Could you check a few things on this model? Use its own coordinates, in mm. A direction names the side the tool comes from. Give positions to 0.01 mm unless a question says otherwise; leave off trailing zeros. Write each loop counter-clockwise with the first axis right and the second up, starting at its lowest first coordinate (ties: lowest second). Pieces come first, ordered by that corner, then holes. Notation, with made-up numbers: M 83.5,28.25 L 103.5,28.25 A17 cw 103.5,36.25 Z; hole C 3,40 d1. An arc over 180 degrees is marked long. Write each question's results on one line, items separated by ' | '. Start each with the question number.
from build123d import *

# Parameters (mm, degrees)
F0_W          = 15.875
F0_H          = 50.8
F1_DEPTH      = 6.35
F2_W          = 31.75
F2_H          = 8.6
F2_R          = 1.75
F3_DEPTH      = 3.175
F3_DEPTH_BACK = 6.35
F4_R          = 4.7625
F5_DEPTH      = 2.54
F6_SIZE       = 2.54
F8_DEPTH      = 5.08
F9_R          = 3.81
F11_DEPTH     = 3.175
F12_SIZE      = 3.17499


# Not quite as in the source:
# - a fillet or chamfer is up to 0.001 mm smaller than in the source, because OpenCascade refuses the exact size


with BuildPart() as f1:
    # F0 (on Top) → F1 (new body)
    with BuildSketch(Plane.XY):
        Rectangle(F0_W, F0_H)
        with BuildLine():
            ThreePointArc((-3.175, -18.058110271), (0.0514516208, -14.8835271912), (3.1733324288, -18.161))
            Line((3.1733324288, -18.161), (3.1733324288, -19.431))
            ThreePointArc((3.1733324288, -19.431), (-0.053119192, -22.6055830798), (-3.175, -19.328110271))
            Line((-3.175, -19.328110271), (-3.175, -18.058110271))
        make_face(mode=Mode.SUBTRACT)
        with BuildLine():
            ThreePointArc((3.1733324288, 18.161), (0.0514516208, 14.8835271912), (-3.175, 18.058110271))
            Line((-3.175, 18.058110271), (-3.175, 19.328110271))
            ThreePointArc((-3.175, 19.328110271), (-0.053119192, 22.6055830798), (3.1733324288, 19.431))
            Line((3.1733324288, 19.431), (3.1733324288, 18.161))
        make_face(mode=Mode.SUBTRACT)
    extrude(amount=F1_DEPTH)

    # F2 (on face) → F3 (join, two sides)
    with BuildSketch(Plane.XY.offset(6.35)) as f3_sk:
        with Locations((0, 9.525)):
            Rectangle(F2_W, F2_H)
        with Locations((-10.795, 9.525)):
            Circle(F2_R, mode=Mode.SUBTRACT)
        with Locations((10.795, 9.525)):
            Circle(F2_R, mode=Mode.SUBTRACT)
    extrude(amount=F3_DEPTH)
    extrude(f3_sk.sketch, amount=-F3_DEPTH_BACK)

    # F4 (on face) → F5 (cut)
    with BuildSketch(Plane.XY.offset(6.35)):
        with Locations((0, -18.796)):
            Circle(F4_R)
        with Locations((0, 18.796)):
            Circle(F4_R)
    extrude(amount=-F5_DEPTH, mode=Mode.SUBTRACT)

    # F6
    f6_edges = [f1.edges().sort_by_distance(p)[0] for p in [
        (-15.875, 9.525, 0),
        (15.875, 9.525, 0),
    ]]
    chamfer(f6_edges, length=F6_SIZE)

    # F7 (on face) → F8 (cut)
    with BuildSketch(Plane(origin=(0, 0, 0), x_dir=(1, 0, 0), z_dir=(0, 0, -1))):
        Polygon((-9.1818833479, -12.319), (-7.5687666958, -9.525), (-9.1818833479, -6.731), (-12.4081166521, -6.731), (-14.0212333042, -9.525), (-12.4081166521, -12.319), align=None)
        Polygon((12.4081166521, -6.731), (9.1818833479, -6.731), (7.5687666958, -9.525), (9.1818833479, -12.319), (12.4081166521, -12.319), (14.0212333042, -9.525), align=None)
    extrude(amount=-F8_DEPTH, mode=Mode.SUBTRACT)

    # F9
    f9_edges = [f1.edges().sort_by_distance(p)[0] for p in [
        (-7.9375, 5.225, 3.175),
        (7.9375, 5.225, 3.175),
        (7.9375, 13.825, 3.175),
        (-7.9375, 13.825, 3.175),
    ]]
    fillet(f9_edges, radius=F9_R)

    # F10 (on face) → F11 (join, through all)
    with BuildSketch(Plane.XY.offset(6.35)):
        with BuildLine():
            Line((-5, 5.225), (-7.6321601122, 5.225))
            Line((-7.6321601122, 5.225), (-1.2342699774, -14.1962191495))
            ThreePointArc((-1.2342699774, -14.1962191495), (0, -14.0335), (1.2342699774, -14.1962191495))
            Line((1.2342699774, -14.1962191495), (7.6321601122, 5.225))
            Line((7.6321601122, 5.225), (5, 5.225))
            Line((5, 5.225), (0, -9.952831082))
            Line((0, -9.952831082), (-5, 5.225))
        make_face()
    extrude(amount=F11_DEPTH)

    # F12 (size 3.175 in the source; OpenCascade refuses exactly that, so slightly less here)
    f12_edges = [f1.edges().sort_by_distance(p)[0] for p in [
        (0, -14.0335, 9.525),
    ]]
    chamfer(f12_edges, length=F12_SIZE)


solid = f1.part
Q1. If we section it at A-A (x = -10.5): Please give me the cut outline in (y, z) (3 decimals), plus the area to 3 significant figures.
Q2. If we mould it in two halves opening along X, with no side actions, what happens to faces 1 (the face through (14.587, 9.465, 1.252)), 2 (the face through (-9.083, 4.139, 3.219)), 3 (the face through (12, 11, 5.08))? For each: pulls with the +X half, pulls with the -X half, needs draft (parallel to the pull), parting line crosses it, or undercut.
Q3. I'm going to push flat-ended pins straight in: P1, Ø1, axis at x = -10, z = 2, coming from the +Y side; P2, Ø1.4, axis at y = -18.5, z = 2.5, coming from the -X side; P3, Ø2, axis at x = 1, y = 2, coming from the +Z side; P4, Ø3, axis at x = -10.795, y = 9.525, coming from the +Z side. Where does each tip first touch, or does it pass through?
Q4. For faces 4 (the face through (-3.175, -19, 2)), 5 (the face through (-4.478, -4.35, 7.915)), 6 (the face through (-7.938, 21, 3)), which set-ups out of +Z, -Z, +X, -X, +Y, -Y let a thin tool reach every point of the face, with its end or its side?
Q5. Please list where these lines run through material, in increasing order: line 1 (Y direction, x = 0, z = 4.5); line 2 (Y direction, x = -12, z = 2.75) (3 decimals); line 3 (Z direction, x = 6, y = -19). Write a range as [from, to].
Q6. If we section it at B-B (y = 21.5): Please give me the cut outline in (x, z).
Determined:
1) outline: M 5.015,0 L 6.731,0 L 6.731,5.08 L 7.8,5.08 L 7.8,9.525 L 5.225,9.525 L 5.225,6.35 L 5.015,6.35 Z; M 11.25,5.08 L 12.319,5.08 L 12.319,0 L 14.035,0 L 14.035,6.35 L 13.825,6.35 L 13.825,9.525 L 11.25,9.525 Z | area: 40.9 mm²
2) face 1: pulls with the +X half | face 2: pulls with the -X half | face 3: undercut
3) P1: stops at y = 14.56 | P2: stops at x = -7.94 | P3: stops at z = 6.35 | P4: passes through
4) face 4: +Z, -Z | face 5: +Z, -X, -Y | face 6: +Z, -Z, -X, +Y
5) line 1: y = [-25.4, -23.56], [-14.03, 14.03], [23.56, 25.4] | line 2: y = [5.225, 6.731], [12.319, 13.825] | line 3: z = [0, 6.35]
6) outline: M -7.94,0 L -2.41,0 L -2.41,3.81 L -3.92,3.81 L -3.92,6.35 L -7.94,6.35 Z; M 2.41,0 L 7.94,0 L 7.94,6.35 L 3.92,6.35 L 3.92,3.81 L 2.41,3.81 Z
